Could you check a few things on this model? Use its own coordinates, in mm. Face numbers are marked on the shaded views. A direction names the side the tool comes from. Round coordinates to 2 decimals unless told otherwise and drop trailing zeros. Loops run counter-clockwise (first coordinate to the right, second up) from the corner with the lowest first, then second, coordinate; pieces in that order, holes last. Notation, with made-up numbers: (-9, 87) - (0, 87) arc R26 ccw to (0, 117) - close; hole circle Ø9 at (-21.5, 66). An arc over 180 degrees is marked (long way). Answer as CSV lines item,"result". Start each with the question number.
1) I'm going to push flat-ended pins straight in: pin 1 Ø4 at (x, y) = (-5, 24.75) entering from +Z; pin 2 Ø1 at (x, z) = (-5.5, 27) entering from -Y; pin 3 Ø1.5 at (x, y) = (3.5, 15) entering from +Z; pin 4 Ø3.5 at (x, y) = (-1, 22.5) entering from +Z. Where does each tip first touch, or does it pass through?
2) Suppose I cut it at C-C, the plane x = 0. Write out the boundary of the cut face in (y, z).
3) Suppose I cut it at B-B, the plane y = -24.75. Write out the boundary of the cut face in (x, z).
4) Please list where these lines run through material, in increasing order: line 1 along Y through (x, z) = (5, 29); line 2 along X through (y, z) = (24, 29); line 3 along X through (y, z) = (23, 28.5).
5) Which directions (+Z, -Z, +X, -X, +Y, -Y) give clear straight access to the entire face, cutting with the end or side of a thin tool? Please do the marked faces 1, 2 and 3.
6) Suppose I cut it at A-A, the plane x = 5. Write out the boundary of the cut face in (y, z).
7) Suppose I cut it at D-D, the plane z = 24. Write out the boundary of the cut face in (x, y), then the cut area to 3 significant figures.
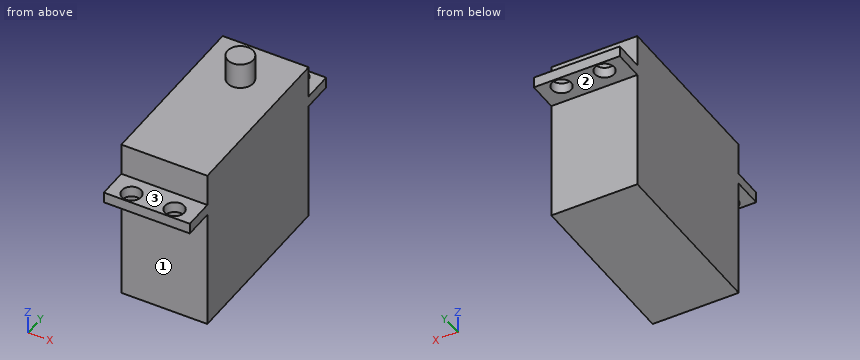
```python
from build123d import *

# Parameters (mm, degrees)
F0_W     = 20
F0_H     = 40.5
F1_DEPTH = 38.1
F3_START = 28.1
F2_W     = 20
F2_H     = 54.5
F3_DEPTH = 2.5
F4_R     = 2.25
F5_DEPTH = 2.5
F6_R     = 3
F7_DEPTH = 6


with BuildPart() as f1:
    # F0 (on Top) → F1 (new body)
    with BuildSketch(Plane.XY):
        Rectangle(F0_W, F0_H)
    extrude(amount=F1_DEPTH)

    # F2 (on Top) → F3 (join)
    with BuildSketch(Plane.XY.offset(F3_START)):
        Rectangle(F2_W, F2_H)
    extrude(amount=F3_DEPTH)

    # F4 (on face) → F5 (cut)
    with BuildSketch(Plane.XY.offset(30.6)):
        with Locations((-5, 24.75)):
            Circle(F4_R)
        with Locations((5, 24.75)):
            Circle(F4_R)
        with Locations((5, -24.75)):
            Circle(F4_R)
        with Locations((-5, -24.75)):
            Circle(F4_R)
    extrude(amount=-F5_DEPTH, mode=Mode.SUBTRACT)

    # F6 (on face) → F7 (join)
    with BuildSketch(Plane.XY.offset(38.1)):
        with Locations((0, 10.15)):
            Circle(F6_R)
    extrude(amount=F7_DEPTH)


solid = f1.part
```
Filled sheet:
1,pin 1,"through"
1,pin 2,"y = -20.25"
1,pin 3,"z = 38.1"
1,pin 4,"z = 30.6"
2,outline,"(-27.25, 28.1) - (-20.25, 28.1) - (-20.25, 0) - (20.25, 0) - (20.25, 28.1) - (27.25, 28.1) - (27.25, 30.6) - (20.25, 30.6) - (20.25, 38.1) - (13.15, 38.1) - (13.15, 44.1) - (7.15, 44.1) - (7.15, 38.1) - (-20.25, 38.1) - (-20.25, 30.6) - (-27.25, 30.6) - close"
3,outline,"(-10, 28.1) - (-7.25, 28.1) - (-7.25, 30.6) - (-10, 30.6) - close; (-2.75, 28.1) - (2.75, 28.1) - (2.75, 30.6) - (-2.75, 30.6) - close; (7.25, 28.1) - (10, 28.1) - (10, 30.6) - (7.25, 30.6) - close"
4,line 1,"-27.25 to -27, -22.5 to 22.5, 27 to 27.25"
4,line 2,"-10 to -7.12, -2.88 to 2.88, 7.12 to 10"
4,line 3,"-10 to -6.41, -3.59 to 3.59, 6.41 to 10"
5,face 1,"-Z, +X, -X, -Y"
5,face 2,"-Z, +X, -X, +Y"
5,face 3,"+Z, +X, -X, -Y"
6,outline,"(-27.25, 28.1) - (-27, 28.1) - (-27, 30.6) - (-27.25, 30.6) - close; (-22.5, 28.1) - (-20.25, 28.1) - (-20.25, 0) - (20.25, 0) - (20.25, 28.1) - (22.5, 28.1) - (22.5, 30.6) - (20.25, 30.6) - (20.25, 38.1) - (-20.25, 38.1) - (-20.25, 30.6) - (-22.5, 30.6) - close; (27, 28.1) - (27.25, 28.1) - (27.25, 30.6) - (27, 30.6) - close"
7,outline,"(-10, -20.25) - (10, -20.25) - (10, 20.25) - (-10, 20.25) - close"
7,area,"810 mm²"
